Could you check a few things on this model? Use its own coordinates, in mm. Face numbers are marked on the shaded views. A direction names the side the tool comes from. Round coordinates to 2 decimals unless told otherwise and drop trailing zeros. Order: outer loops, then holes, each group sorted by start corner. A loop starts at its lowest first (then second) coordinate and runs counter-clockwise, first axis right, second up. Notation, with made-up numbers: (-31, 82) - (15, 82) arc R24 cw to (15, 108) - close; hole circle Ø7 at (-14, 84.25). An arc over 180 degrees is marked (long way). Use one line per item in the form item = value.
from build123d import *

# Parameters (mm, degrees)
SKETCH1_R           = 7.62
BOSS_EXTRUDE1_DEPTH = 25.4
SKETCH3_R           = 3.81
BOSS_EXTRUDE2_DEPTH = 2.54
SKETCH4_R           = 3.81
BOSS_EXTRUDE3_DEPTH = 2.54


with BuildPart() as part:
    # Sketch1 → Boss-Extrude1 (new body)
    with BuildSketch(Plane.XY):
        Circle(SKETCH1_R)
    extrude(amount=BOSS_EXTRUDE1_DEPTH)

    # Cut-Sweep1: sweep along a curve in space
    with BuildLine() as cut_sweep1_path:
        ThreePointArc((7.62, 0, 0), (5.388153673, 5.388153673, 0), (0, 7.62, 0))
        ThreePointArc((0, 7.62, 0), (-5.388153673, 5.388153673, 0), (-7.62, 0, 0))
        ThreePointArc((-7.62, 0, 0), (-5.388153673, -5.388153673, 0), (0, -7.62, 0))
        ThreePointArc((0, -7.62, 0), (5.388153673, -5.388153673, 0), (7.62, 0, 0))
    # Sketch2 → Cut-Sweep1 (sweep, cut)
    with BuildSketch(Plane(origin=(0, 0, 0), x_dir=(1, 0, 0), z_dir=(0, 1, 0))):
        with BuildLine():
            Line((7.62, -9.950369343), (7.62, -15.449630657))
            ThreePointArc((7.62, -15.449630657), (6.0325, -12.7), (7.62, -9.950369343))
        make_face()
    sweep(path=cut_sweep1_path.line, mode=Mode.SUBTRACT)

    # Sketch3 → Boss-Extrude2 (add)
    with BuildSketch(Plane.XY.offset(25.4)):
        Circle(SKETCH3_R)
    extrude(amount=BOSS_EXTRUDE2_DEPTH)

    # Sketch4 → Boss-Extrude3 (add)
    with BuildSketch(Plane(origin=(0, 0, 0), x_dir=(-1, 0, 0), z_dir=(0, 0, -1))):
        with Locations(Location((0, 0, 0), (0, 0, 180))):
            Circle(SKETCH4_R)
    extrude(amount=BOSS_EXTRUDE3_DEPTH)


solid = part.part
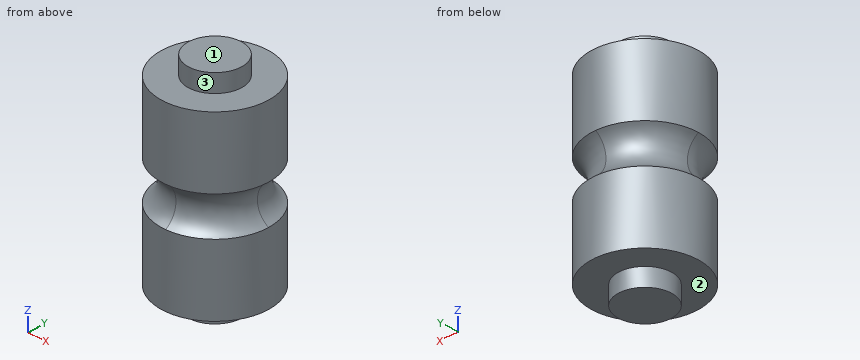
Item 1: For the marked faces 1, 2 and 3, which set-ups out of +Z, -Z, +X, -X, +Y, -Y let a thin tool reach every point of the face, with its end or its side?
Found:
face_1 = +Z, +X, -X, +Y, -Y
face_2 = -Z
face_3 = +Z
Item 2: Imagine slicing it at A-A on z = 20. Please give me the cut outline in (x, y).
Found:
outline = circle Ø15.24 at (0, 0)
Item 3: I need wall thicknesses on L1, parallel to Z at x = 2, y = -3.5; L2, parallel to Z at x = 4.5, y = -4.5; L3, parallel to Z at x = 2, y = -7. Which ranges of each line are inside material? Lowest first, please.
Found:
L1 = 0 to 25.4
L2 = 0 to 11.29, 14.11 to 25.4
L3 = 0 to 10.18, 15.22 to 25.4
Item 4: Will these pins go through, and if not, where does the flat tip stop? P1, Ø2, axis at x = -2.5, z = 4.5, coming from the -Y side; P2, Ø1.5, axis at x = -4.5, z = 16.5, coming from the +Y side; P3, Ø2, axis at y = -1.5, z = 11.5, coming from the +X side.
Found:
P1 = -7.47
P2 = 6.63
P3 = 6.78
